Could you check a few things on this model? Use its own coordinates, in mm. Round coordinates to 2 decimals unless told otherwise and drop trailing zeros. Write each loop counter-clockwise with the first axis right and the second up, starting at its lowest first coordinate (ties: lowest second). Pieces come first, ordered by that corner, then holes. Notation, with made-up numbers: (34.5, -8) -> (62.5, -8) arc R23 ccw to (62.5, 6) -> close; hole circle Ø8 at (37.25, 59.5). An arc over 180 degrees is marked (long way). Answer as CSV lines item,"result". Start each with the question number.
Q1. Imagine slicing it at C-C on y = 3.25. Please give me the cut outline in (x, z).
Q2. Imagine slicing it at B-B on z = 0. Please give me the cut outline in (x, y).
Q3. Imagine slicing it at A-A on x = 0. Please give me the cut outline in (y, z), and give its area (3 significant figures).
Q4. If I drill on line 1 (Z direction, x = 0, y = 3.2); line 2 (X direction, y = 3.5, z = 0); line 3 (Z direction, x = 34.5, y = 4.25), over which ranges is the centre line in solid material (lowest first)? Write a range as [from, to].
Q5. Imagine slicing it at D-D on x = 17. Please give me the cut outline in (y, z).
Q6. Will these pins go through, and if not, where does the flat tip stop? pin 1 Ø2 at (x, y) = (52.5, 3) entering from +Z; pin 2 Ø3 at (y, z) = (3.5, -42) entering from -X; pin 3 Ø1.5 at (x, y) = (-50.5, 1) entering from -Z.
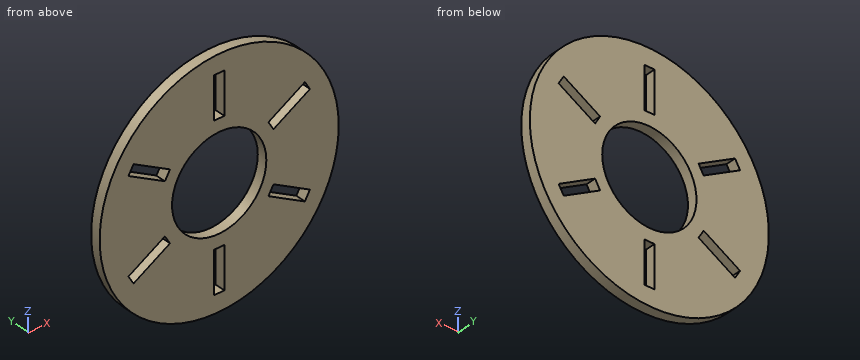
from build123d import *

# Parameters (mm, degrees)
ESQUISSE1_R             = 71
ESQUISSE1_R_2           = 28
BOSS_EXTRU_1_DEPTH      = 6
ESQUISSE2_W             = 6
ESQUISSE2_H             = 25
ENL_V_MAT_EXTRU_1_DEPTH = 10


with BuildPart() as part:
    # Esquisse1 → Boss.-Extru.1 (new body)
    with BuildSketch(Plane(origin=(0, 0, 0), x_dir=(1, 0, 0), z_dir=(0, 1, 0))):
        Circle(ESQUISSE1_R)
        Circle(ESQUISSE1_R_2, mode=Mode.SUBTRACT)
    extrude(amount=BOSS_EXTRU_1_DEPTH)

    # Esquisse2 → Enlèv. mat.-Extru.1 (cut)
    with BuildSketch(Plane.XZ):
        Polygon((50.894536929, -32.848076211), (29.243901834, -20.348076211), (32.243901834, -15.151923789), (53.894536929, -27.651923789), align=None)
        with Locations((0, -48)):
            Rectangle(ESQUISSE2_W, ESQUISSE2_H)
        Polygon((53.894536929, 27.651923789), (32.243901834, 15.151923789), (29.243901834, 20.348076211), (50.894536929, 32.848076211), align=None)
        with Locations((0, 48)):
            Rectangle(ESQUISSE2_W, ESQUISSE2_H)
        Polygon((-50.894536929, 32.848076211), (-29.243901834, 20.348076211), (-32.243901834, 15.151923789), (-53.894536929, 27.651923789), align=None)
        Polygon((-53.894536929, -27.651923789), (-32.243901834, -15.151923789), (-29.243901834, -20.348076211), (-50.894536929, -32.848076211), align=None)
    extrude(amount=-ENL_V_MAT_EXTRU_1_DEPTH, mode=Mode.SUBTRACT)


solid = part.part
Checks:
1,outline,"circle Ø142 at (0, 0); hole (-53.89, -27.65) -> (-50.89, -32.85) -> (-29.24, -20.35) -> (-32.24, -15.15) -> close; hole (-53.89, 27.65) -> (-32.24, 15.15) -> (-29.24, 20.35) -> (-50.89, 32.85) -> close; hole circle Ø56 at (0, 0); hole (-3, -60.5) -> (3, -60.5) -> (3, -35.5) -> (-3, -35.5) -> close; hole (-3, 35.5) -> (3, 35.5) -> (3, 60.5) -> (-3, 60.5) -> close; hole (29.24, -20.35) -> (50.89, -32.85) -> (53.89, -27.65) -> (32.24, -15.15) -> close; hole (29.24, 20.35) -> (32.24, 15.15) -> (53.89, 27.65) -> (50.89, 32.85) -> close"
2,outline,"(-71, 0) -> (-28, 0) -> (-28, 6) -> (-71, 6) -> close; (28, 0) -> (71, 0) -> (71, 6) -> (28, 6) -> close"
3,outline,"(0, -71) -> (6, -71) -> (6, -60.5) -> (0, -60.5) -> close; (0, -35.5) -> (6, -35.5) -> (6, -28) -> (0, -28) -> close; (0, 28) -> (6, 28) -> (6, 35.5) -> (0, 35.5) -> close; (0, 60.5) -> (6, 60.5) -> (6, 71) -> (0, 71) -> close"
3,area,"216 mm^2"
4,line 1,"[-71, -60.5], [-35.5, -28], [28, 35.5], [60.5, 71]"
4,line 2,"[-71, -28], [28, 71]"
4,line 3,"[-62.05, -23.38], [-16.45, 16.45], [23.38, 62.05]"
5,outline,"(0, -68.93) -> (6, -68.93) -> (6, -22.25) -> (0, -22.25) -> close; (0, 22.25) -> (6, 22.25) -> (6, 68.93) -> (0, 68.93) -> close"
6,pin 1,"z = 48.87"
6,pin 2,"x = -58.32"
6,pin 3,"z = -50.66"
